Input: dimensioned drawing with shaded views. Units: mm. Origin: part minimum x, y, z. A direction names the side the tool comes from. Give positions to 0.01 mm unless a question says otherwise; leave off trailing zeros. Write each loop counter-clockwise with the first axis right and the second up, starting at its lowest first coordinate (ties: lowest second). Pieces come first, ordered by that corner, then holes.
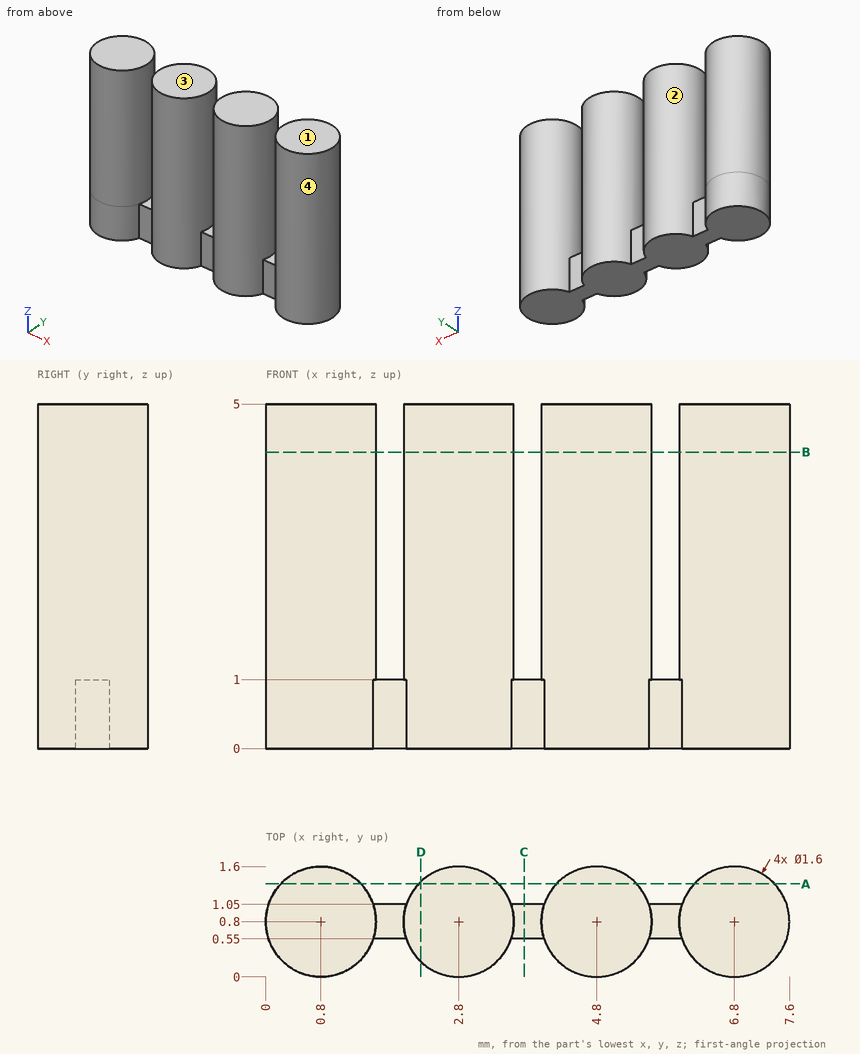
Item 1: Section D-D (x = 2.25). Return loops of the section in (y, z).
Item 2: Ray query, line 1 (X direction, y = 0.15, z = 1.7); line 2 (X direction, y = 1.1, z = 1.05); line 3 (Y direction, x = 4.75, z = 4.6). Return the intervals inside material, ascending.
Item 3: Section B-B (z = 4.3). Return loops of the section in (x, y).
Item 4: Section C-C (x = 3.75). Return loops of the section in (y, z).
Item 5: Set-up query: the marked faces 1 and 2. Return all of +Z, -Z, +X, -X, +Y, -Y with unobstructed straight access to the full face (end or side cutting, diameter ignored); none if empty.
Item 6: Section A-A (y = 1.35). Return loops of the section in (x, z), and give its area (3 significant figures).
Item 7: Mould query, pull axis X, two halves, no side actions, for the marked faces 3 and 4. Classes: +X half, -X half, draft (parallel to the pull), parting line (faces both ways), or undercut.
Solved:
1. outline: (0.22, 0) - (1.38, 0) - (1.38, 5) - (0.22, 5) - close
2. line 1: x = 0.33 to 1.27, 2.33 to 3.27, 4.33 to 5.27, 6.33 to 7.27
2. line 2: x = 0.06 to 1.54, 2.06 to 3.54, 4.06 to 5.54, 6.06 to 7.54
2. line 3: y = 0 to 1.6
3. outline: circle Ø1.6 at (0.8, 0.8); circle Ø1.6 at (2.8, 0.8); circle Ø1.6 at (4.8, 0.8); circle Ø1.6 at (6.8, 0.8)
4. outline: (0.55, 0) - (1.05, 0) - (1.05, 1) - (0.55, 1) - close
5. face 1: +Z, +X, -X, +Y, -Y
5. face 2: +Z
6. outline: (0.22, 0) - (1.38, 0) - (1.38, 5) - (0.22, 5) - close; (2.22, 0) - (3.38, 0) - (3.38, 5) - (2.22, 5) - close; (4.22, 0) - (5.38, 0) - (5.38, 5) - (4.22, 5) - close; (6.22, 0) - (7.38, 0) - (7.38, 5) - (6.22, 5) - close
6. area: 23.2 mm2
7. face 3: draft
7. face 4: undercut
